The listing builds one solid part. Answer for the finished solid, in the listing's coordinates (mm). Face numbers are marked on the shaded views. A direction names the side the tool comes from. Give positions to 0.01 mm unless a question says otherwise; leave off trailing zeros. Write each loop counter-clockwise with the first axis right and the second up, starting at its lowest first coordinate (ties: lowest second). Pieces come first, ordered by that corner, then holes. Notation, with made-up numbers: (64.5, 47.25) - (77.5, 47.25) arc R20 ccw to (77.5, 57.25) - close; hole circle Ø3 at (-9, 80). An arc over 180 degrees is marked (long way). Return JSON: item names as keys, results as strings.
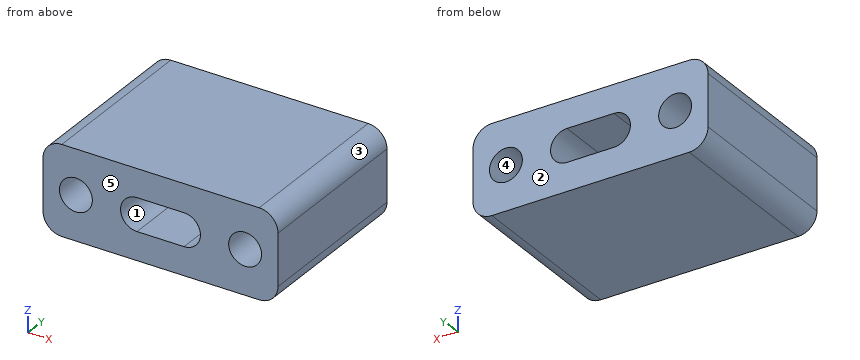
from build123d import *

# Parameters (mm, degrees)
SKETCH_1_W      = 25
SKETCH_1_H      = 9.5
SKETCH_1_R      = 1.75
EXTRUDE_1_DEPTH = 18
FILLET_1_R      = 2


with BuildPart() as part:
    # 草图1 → 凸台-拉伸1 (new body)
    with BuildSketch(Plane(origin=(0, 0, 0), x_dir=(1, 0, 0), z_dir=(0, 1, 0))):
        Rectangle(SKETCH_1_W, SKETCH_1_H)
        with Locations(Location((-9, 0, 0), (0, 0, 270))):
            Circle(SKETCH_1_R, mode=Mode.SUBTRACT)
        with Locations(Location((9, 0, 0), (0, 0, 270))):
            Circle(SKETCH_1_R, mode=Mode.SUBTRACT)
        with BuildLine():
            Line((-2.5, 1.75), (2.5, 1.75))
            ThreePointArc((2.5, 1.75), (4.25, 0), (2.5, -1.75))
            Line((2.5, -1.75), (-2.5, -1.75))
            ThreePointArc((-2.5, -1.75), (-4.25, 0), (-2.5, 1.75))
        make_face(mode=Mode.SUBTRACT)
    extrude(amount=EXTRUDE_1_DEPTH)

    # 圆角1
    fillet_1_edges = [part.edges().sort_by_distance(p)[0] for p in [
        (12.5, 9, 4.75),
        (-12.5, 9, 4.75),
        (-12.5, 9, -4.75),
        (12.5, 9, -4.75),
    ]]
    fillet(fillet_1_edges, radius=FILLET_1_R)


solid = part.part
Item 1: A cutting plane is placed at C-C on x = 9. Determine the outline of the cut face in (y, z).
Answer below:
{"outline": "(0, -4.75) - (18, -4.75) - (18, -1.75) - (0, -1.75) - close; (0, 1.75) - (18, 1.75) - (18, 4.75) - (0, 4.75) - close"}
Item 2: Consider L1, parallel to X at y = 10.5, z = 0; L2, parallel to X at y = 13, z = -0.75; L3, parallel to Z at x = 10.25, y = 6.75. Determine where each line is inside the solid, lowest interval first.
Answer below:
{"L1": "x = -12.5 to -10.75, -7.25 to -4.25, 4.25 to 7.25, 10.75 to 12.5", "L2": "x = -12.5 to -10.58, -7.42 to -4.08, 4.08 to 7.42, 10.58 to 12.5", "L3": "z = -4.75 to -1.22, 1.22 to 4.75"}
Item 3: The mould has two halves that part along X. Classify the marked faces 3, 4 and 5: +X half, -X half, draft (parallel to the pull), parting line (faces both ways), or undercut.
Answer below:
{"face 3": "+X half", "face 4": "undercut", "face 5": "draft"}
Item 4: A cutting plane is placed at B-B on z = 0. Determine the outline of the cut face in (x, y).
Answer below:
{"outline": "(-12.5, 0) - (-10.75, 0) - (-10.75, 18) - (-12.5, 18) - close; (-7.25, 0) - (-4.25, 0) - (-4.25, 18) - (-7.25, 18) - close; (4.25, 0) - (7.25, 0) - (7.25, 18) - (4.25, 18) - close; (10.75, 0) - (12.5, 0) - (12.5, 18) - (10.75, 18) - close"}
Item 5: A cutting plane is placed at D-D on x = -7.75. Determine the outline of the cut face in (y, z).
Answer below:
{"outline": "(0, -4.75) - (18, -4.75) - (18, -1.22) - (0, -1.22) - close; (0, 1.22) - (18, 1.22) - (18, 4.75) - (0, 4.75) - close"}
Item 6: For the marked faces 1 and 2, determine the directions among +Z, -Z, +X, -X, +Y, -Y from which every point of the face is accessible in a straight line to the end or side of a thin tool.
Answer below:
{"face 1": "+Y, -Y", "face 2": "+Z, -Z, +X, -X, +Y"}
Item 7: A cutting plane is placed at A-A on y = 7. Determine the outline of the cut face in (x, z).
Answer below:
{"outline": "(-12.5, -2.75) arc R2 ccw to (-10.5, -4.75) - (10.5, -4.75) arc R2 ccw to (12.5, -2.75) - (12.5, 2.75) arc R2 ccw to (10.5, 4.75) - (-10.5, 4.75) arc R2 ccw to (-12.5, 2.75) - close; hole circle Ø3.5 at (-9, 0); hole (-2.5, -1.75) - (2.5, -1.75) arc R1.75 ccw to (2.5, 1.75) - (-2.5, 1.75) arc R1.75 ccw to start; hole circle Ø3.5 at (9, 0)"}
Item 8: A flat-ended cylindrical pin translates along its axis: P1, Ø1, axis at x = -4.5, z = -1, coming from the -Y side. Find the tip coordinate at first contact, or state that the pin passes through.
Answer below:
{"P1": "stops at y = 0"}
